Here's how the part is built. I have some questions about the finished solid (model axes, mm). A direction names the side the tool comes from. Coordinates: 2 decimals unless noted, no trailing zeros. Order: outer loops, then holes, each group sorted by start corner. A loop starts at its lowest first (then second) coordinate and runs counter-clockwise, first axis right, second up. Notation, with made-up numbers: (-26, -24) - (24, -24) arc R20 ccw to (24, 11) - close; hole circle Ø10 at (2, 44). An arc over 180 degrees is marked (long way). Answer as CSV lines item,"result". Start each with the question number.
Item 1: We'd pull the mould along Z, two halves only. Please class faces 1 (the face through (-5, 2, -30)), 2 (the face through (1.981, 2.535, -51.974)), 3 (the face through (25, -24, -40)): pulls with the +Z half, pulls with the -Z half, needs draft (parallel to the pull), parting line crosses it, or undercut.
Item 2: Imagine slicing it at C-C on z = -25. List the corners of the cut face in (x, y) for me.
Item 3: I'm going to push flat-ended pins straight in: pin 1 (10 mm diameter, centred on y = -1, z = -22.5, fed in from +X); pin 2 (6 mm diameter, centred on x = 35, y = -15.5, fed in from +Z); pin 3 (8 mm diameter, centred on x = 5, z = -26, fed in from -Y); pin 4 (10 mm diameter, centred on y = -32, z = -31, fed in from -X). Where does each tip first touch, or does it pass through?
Item 4: I need wall thicknesses on line 1 (X direction, y = 2.85, z = -6.5); line 2 (Z direction, x = 1, y = 3); line 3 (X direction, y = 2, z = -6). Which ranges of each line are inside material? Lowest first, please.
Item 5: Imagine slicing it at A-A on x = 48.5. List the corners of the cut face in (y, z) for me, and give its area (3 significant figures).
Item 6: Imagine slicing it at D-D on x = 23. List the corners of the cut face in (y, z) for me.
Item 7: On a 3-axis mill with a long thin cutter (end or side, diameter ignored), from which of +Z, -Z, +X, -X, +Y, -Y can I reach the whole of each face in a straight line? I mean faces 4 (the face through (25, -24, -20)), 5 (the face through (35, -24, -30)), 6 (the face through (15, -24, -30)). Say none if no direction works.
Item 8: Imagine slicing it at B-B on z = -6.5. List the corners of the cut face in (x, y) for me, and give its area (3 significant figures).
from build123d import *

# Parameters (mm, degrees)
SKIZZE1_W                       = 60
SKIZZE1_H                       = 60
AUFSATZ_LINEAR_AUSTRAGEN1_DEPTH = 5
SKIZZE7_R                       = 1.6
SCHNITT_LINEAR_AUSTRAGEN1_DEPTH = 10
FASE1_SIZE                      = 0.5
SKIZZE8_W                       = 20
SKIZZE8_H                       = 20
AUFSATZ_LINEAR_AUSTRAGEN2_DEPTH = 48


with BuildPart() as part:
    # Skizze1 → Aufsatz-Linear austragen1 (new body)
    with BuildSketch(Plane(origin=(0, 0, 0), x_dir=(1, 0, 0), z_dir=(0, 1, 0))):
        with Locations((25, 30)):
            Rectangle(SKIZZE1_W, SKIZZE1_H)
    extrude(amount=AUFSATZ_LINEAR_AUSTRAGEN1_DEPTH)

    # Skizze7 → Schnitt-Linear austragen1 (cut)
    with BuildSketch(Plane(origin=(0, 5, 0), x_dir=(1, 0, 0), z_dir=(0, 1, 0))):
        with Locations(Location((1.5, 53.5, 0), (0, 0, 270))):
            Circle(SKIZZE7_R)
        with Locations(Location((48.5, 53.5, 0), (0, 0, 270))):
            Circle(SKIZZE7_R)
        with Locations(Location((48.5, 6.5, 0), (0, 0, 270))):
            Circle(SKIZZE7_R)
        with Locations(Location((1.5, 6.5, 0), (0, 0, 270))):
            Circle(SKIZZE7_R)
    extrude(amount=-SCHNITT_LINEAR_AUSTRAGEN1_DEPTH, mode=Mode.SUBTRACT)

    # Fase1
    fase1_edges = [part.edges().sort_by_distance(p)[0] for p in [
        (-5, 2.5, -60),
        (55, 2.5, -60),
        (55, 2.5, 0),
        (-5, 2.5, 0),
    ]]
    chamfer(fase1_edges, length=FASE1_SIZE)

    # Skizze8 → Aufsatz-Linear austragen2 (add)
    with BuildSketch(Plane.XZ):
        with Locations((25, -30)):
            Rectangle(SKIZZE8_W, SKIZZE8_H)
    extrude(amount=AUFSATZ_LINEAR_AUSTRAGEN2_DEPTH)


solid = part.part
Responses:
1,face 1,"needs draft"
1,face 2,"undercut"
1,face 3,"pulls with the -Z half"
2,outline,"(-5, 0) - (15, 0) - (15, -48) - (35, -48) - (35, 0) - (55, 0) - (55, 5) - (-5, 5) - close"
3,pin 1,"stops at x = 55"
3,pin 2,"stops at z = -20"
3,pin 3,"stops at y = 0"
3,pin 4,"stops at x = 15"
4,line 1,"x = -5 to -0.1, 3.1 to 46.9, 50.1 to 55"
4,line 2,"z = -60 to -55.02, -51.98 to -8.02, -4.98 to 0"
4,line 3,"x = -5 to -0.02, 3.02 to 46.98, 50.02 to 55"
5,outline,"(0, -60) - (5, -60) - (5, -55.1) - (0, -55.1) - close; (0, -51.9) - (5, -51.9) - (5, -8.1) - (0, -8.1) - close; (0, -4.9) - (5, -4.9) - (5, 0) - (0, 0) - close"
5,area,"268 mm^2"
6,outline,"(-48, -40) - (0, -40) - (0, -60) - (5, -60) - (5, 0) - (0, 0) - (0, -20) - (-48, -20) - close"
7,face 4,"+Z, +X, -X, -Y"
7,face 5,"+Z, -Z, +X, -Y"
7,face 6,"+Z, -Z, -X, -Y"
8,outline,"(-5, 0) - (-0.1, 0) - (-0.1, 5) - (-5, 5) - close; (3.1, 0) - (46.9, 0) - (46.9, 5) - (3.1, 5) - close; (50.1, 0) - (55, 0) - (55, 5) - (50.1, 5) - close"
8,area,"268 mm^2"
